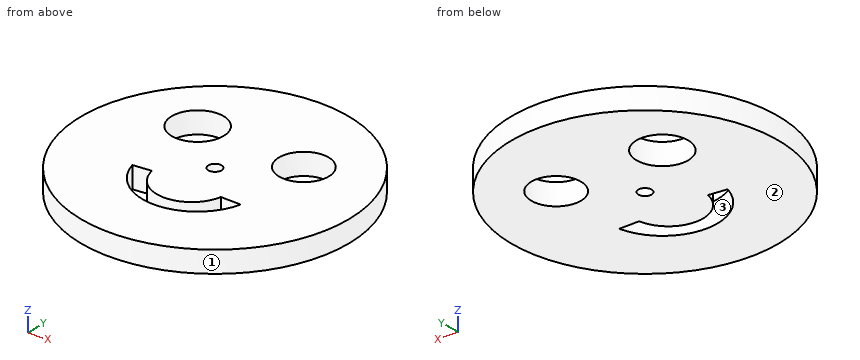
```python
from build123d import *

# Parameters (mm, degrees)
F0_R     = 39.644393
F1_DEPTH = 6.35
F2_R     = 7.676515
F2_R_2   = 7.361152
F2_R_3   = 1.953076
F3_DEPTH = 6.351


with BuildPart() as f1:
    # F0 (on Top) → F1 (new body)
    with BuildSketch(Plane.XY):
        Circle(F0_R)
    extrude(amount=F1_DEPTH)

    # F2 (on face) → F3 (cut, through all)
    with BuildSketch(Plane.XY.offset(6.35)):
        with Locations((-15.738009, 13.301156)):
            Circle(F2_R)
        with Locations((15.738009, 13.098084)):
            Circle(F2_R_2)
        Circle(F2_R_3)
        with BuildLine():
            Line((-10.430831, -10.205741), (-15.738009, -10.814955))
            ThreePointArc((-15.738009, -10.814955), (0.235681, -22.687173), (15.738009, -10.205741))
            Line((15.738009, -10.205741), (9.876276, -10.205741))
            ThreePointArc((9.876276, -10.205741), (-0.277277, -18.591153), (-10.430831, -10.205741))
        make_face()
    extrude(amount=-F3_DEPTH, mode=Mode.SUBTRACT)


solid = f1.part
```
Geometry: final body of the model. Coordinates: model frame, mm. Face numbers are marked on the shaded views. Give positions to 0.01 mm unless a question says otherwise; leave off trailing zeros. Write each loop counter-clockwise with the first axis right and the second up, starting at its lowest first coordinate (ties: lowest second). Pieces come first, ordered by that corner, then holes.
1. Draft query along X for the marked faces 1, 2 and 3. Return one class per face: released by +X, released by -X, zero draft, split by the parting line, or undercut.
2. Section query A-A, the plane y = 0. Return loops of the section in (x, z), then the cut area to 3 significant figures.
3. Section query D-D, the plane z = 4.25. Return loops of the section in (x, y), then the cut area to 3 significant figures.
4. Section query C-C, the plane y = 18. Return loops of the section in (x, z), then the cut area to 3 significant figures.
5. Line query: probe 1 along Y at (x, z) = (0, 2); probe 2 along X at (y, z) = (13.5, 1); probe 3 along Y at (x, z) = (-1.5, 2.25). Output: solid intervals per line, ascending.
6. Pin query (flat end, axial travel): P1, Ø1, axis at x = -26, z = 5, coming from the -Y side; P2, Ø3, axis at x = 12.5, z = 2, coming from the -Y side; P3, Ø1, axis at y = -8, z = 3, coming from the -X side. Return the tip coordinate at first contact, or that it passes through.
7. Section query B-B, the plane x = -1. Return loops of the section in (y, z).
Computed:
1. face 1: split by the parting line
1. face 2: zero draft
1. face 3: undercut
2. outline: (-39.64, 0) - (-1.95, 0) - (-1.95, 6.35) - (-39.64, 6.35) - close; (1.95, 0) - (39.64, 0) - (39.64, 6.35) - (1.95, 6.35) - close
2. area: 479 mm2
3. outline: circle Ø79.29 at (0, 0); hole circle Ø15.35 at (-15.74, 13.3); hole (-15.74, -10.81) arc R16.26 ccw to (15.74, -10.21) - (9.88, -10.21) arc R10.34 cw to (-10.43, -10.21) - close; hole circle Ø3.91 at (0, 0); hole circle Ø14.72 at (15.74, 13.1)
3. area: 4,410 mm2
4. outline: (-35.32, 0) - (-21.81, 0) - (-21.81, 6.35) - (-35.32, 6.35) - close; (-9.67, 0) - (10.25, 0) - (10.25, 6.35) - (-9.67, 6.35) - close; (21.23, 0) - (35.32, 0) - (35.32, 6.35) - (21.23, 6.35) - close
4. area: 302 mm2
5. probe 1: y = -39.64 to -22.69, -18.59 to -1.95, 1.95 to 39.64
5. probe 2: x = -37.28 to -23.41, -8.06 to 8.39, 23.09 to 37.28
5. probe 3: y = -39.62 to -22.63, -18.52 to -1.25, 1.25 to 39.62
6. P1: stops at y = -30.36
6. P2: stops at y = -38.09
6. P3: stops at x = -38.93
7. outline: (-39.63, 0) - (-22.66, 0) - (-22.66, 6.35) - (-39.63, 6.35) - close; (-18.57, 0) - (-1.68, 0) - (-1.68, 6.35) - (-18.57, 6.35) - close; (1.68, 0) - (39.63, 0) - (39.63, 6.35) - (1.68, 6.35) - close
